Input: dimensioned drawing with shaded views. Units: mm. Origin: part minimum x, y, z. A direction names the side the tool comes from. Coordinates: 2 decimals unless noted, no trailing zeros. Loops run counter-clockwise (first coordinate to the right, second up) from the corner with the lowest first, then second, coordinate; pieces in that order, holes last.
Item 1: Reachability of the marked faces 4, 5 and 6 from +Z, -Z, +X, -X, +Y, -Y: full face, straight path, thin tool, end or side. Return the list, or none.
Item 2: Section query A-A, the plane x = 10. Return the cut outline in (y, z), then the cut area to 3 significant figures.
Item 3: Line query: probe 1 along Y at (x, z) = (24, 0.6); probe 2 along X at (y, z) = (33, 2.65); probe 3 along X at (y, z) = (9.5, 4.3) (1 decimal). Output: solid intervals per line, ascending.
Item 4: Pin query (flat end, axial travel): pin 1 Ø1.5 at (y, z) = (49.5, 2) entering from -X (1 decimal); pin 2 Ø1 at (x, z) = (48, 2) entering from +Y; pin 3 Ø1.5 at (y, z) = (49, 3.5) entering from +X (1 decimal). Return the tip coordinate at first contact, or that it passes through.
Item 5: Pull-direction query (Y, two-part tool) for the marked faces 1, 2 and 3; classes: +Y half, -Y half, draft (parallel to the pull), parting line (faces both ways), or undercut.
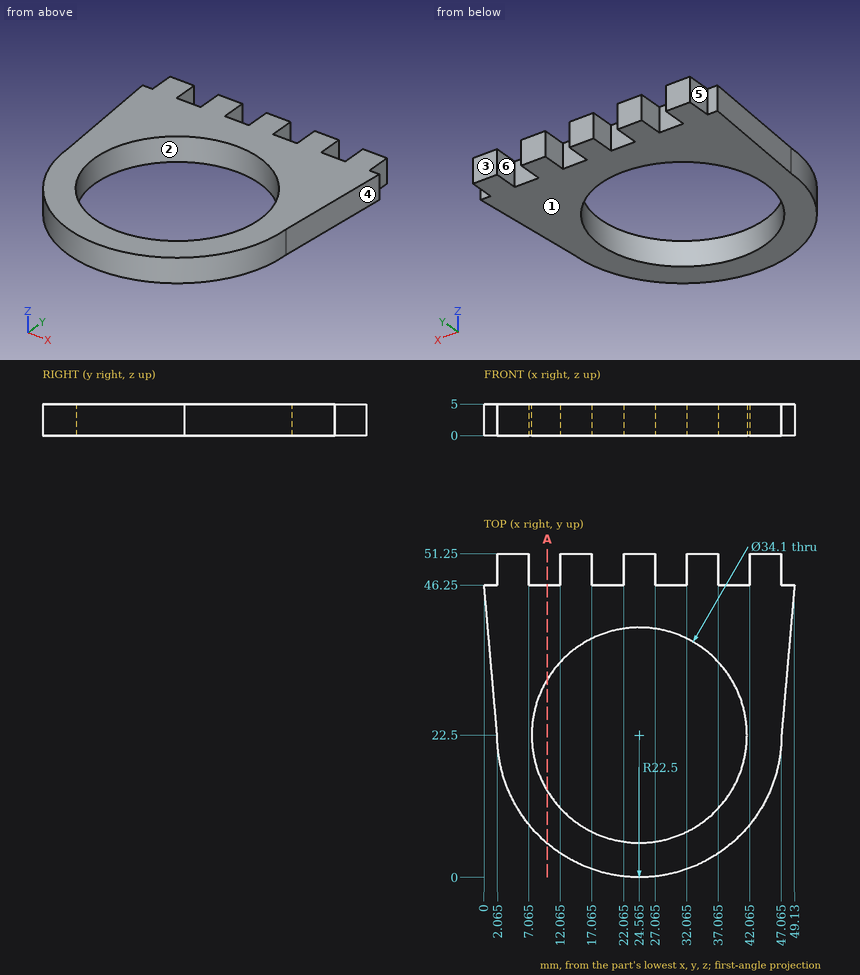
Verdict:
1. face 4: +Z, -Z, +X, -Y
1. face 5: +Z, -Z, -X, +Y
1. face 6: +Z, -Z, +Y
2. outline: (5.35, 0) - (13.64, 0) - (13.64, 5) - (5.35, 5) - close; (31.36, 0) - (46.25, 0) - (46.25, 5) - (31.36, 5) - close
2. area: 116 mm2
3. probe 1: y = 0.01 to 5.46, 39.54 to 51.25
3. probe 2: x = 1.15 to 11.13, 38 to 47.98
3. probe 3: x = 6.2 to 13.5, 35.6 to 42.9
4. pin 1: stops at x = 2.1
4. pin 2: stops at y = 46.25
4. pin 3: stops at x = 47.1
5. face 1: draft
5. face 2: undercut
5. face 3: +Y half
